For this review, take the finished solid that the model builds, in its own axes (mm). A direction names the side the tool comes from. Give positions to 0.01 mm unless a question says otherwise; leave off trailing zeros. Write each loop counter-clockwise with the first axis right and the second up, starting at its lowest first coordinate (ties: lowest second). Pieces come first, ordered by that corner, then holes.
1) We need section A-A on y = 0. Give the boundary of the cut face in (x, z).
2) We need section C-C on x = 0. Give the boundary of the cut face in (y, z).
3) We need section B-B on z = 5.5. Give the boundary of the cut face in (x, y), and give its area (3 significant figures).
4) For P1, Ø4, axis at y = 63.5, z = 3.5, coming from the -X side, flat-tipped, find the tip position at first contact; note if it passes through.
5) Draft analysis for pull direction Y (two halves, no side actions). For faces 3 (the face through (13, 61, 8)), 4 (the face through (1.35, 6.553, 3.944)), 5 (the face through (8.697, 12.384, 4.056)), 6 (the face through (8.712, -0.744, 3.944)), state which applies: pulls with the +Y half, pulls with the -Y half, needs draft (parallel to the pull), parting line crosses it, or undercut.
6) Machinability: for faces 1 (the face through (-4, 123, 4)), 2 (the face through (1.198, 113.535, 3.944)), which of the approach directions +Z, -Z, +X, -X, +Y, -Y give a long, thin tool a straight path to every point of the face, cutting with its end or side? Answer none if there is none.
7) Wall thickness on line 1 along Y through (x, z) = (-0.25, 5.5) (3 decimals); line 2 along Y through (x, z) = (0, 6.25); line 3 along X through (y, z) = (89, 5.25): over which ranges is each line inside the solid? List them lowest first.
from build123d import *

# Parameters (mm, degrees)
SKETCH_1_R          = 5
EXTRUDE_1_DEPTH     = 8
SKETCH_1_R_2        = 5.001260551
EXTRUDE_1_2_DEPTH   = 8
EXTRUDE_4_DEPTH     = 8
SKETCH_5_R          = 2.5
CUT_EXTRUDE_2_DEPTH = 127.842421926
FILLET_1_R          = 10


with BuildPart() as part:
    # Sketch 1 → Extrude 1 (new body)
    with BuildSketch(Plane.XY):
        with Locations((0, 120)):
            Circle(SKETCH_1_R)
    extrude(amount=EXTRUDE_1_DEPTH)



with BuildPart() as body_2:
    # Sketch 1 → Extrude 1 2 (new body)
    with BuildSketch(Plane.XY):
        Circle(SKETCH_1_R_2)
    extrude(amount=EXTRUDE_1_2_DEPTH)


with BuildPart() as part_1:
    add(part.part)

    add(body_2.part)  # Extrude 4 merges body 2
    # Sketch 4 → Extrude 4 (add)
    with BuildSketch(Plane.XY):
        Polygon((-2.5, 115.669872981), (10, 108.452994616), (10, 11.547005384), (-2.5, 4.330127019), (2.5, -4.330127019), (20, 5.773502692), (20, 114.226497308), (2.5, 124.330127019), align=None)
    extrude(amount=EXTRUDE_4_DEPTH)

    # Sketch 5 → Cut-Extrude 2 (cut, through all)
    with BuildSketch(Plane.XY.offset(8)):
        with Locations((0, 120)):
            Circle(SKETCH_5_R)
        Circle(SKETCH_5_R)
    extrude(amount=-CUT_EXTRUDE_2_DEPTH, mode=Mode.SUBTRACT)

    # Fillet 1
    fillet_1_edges = [part_1.edges().sort_by_distance(p)[0] for p in [
        (10, 11.547005384, 4),
        (20, 5.773502692, 4),
        (20, 114.226497308, 4),
        (10, 108.452994616, 4),
    ]]
    fillet(fillet_1_edges, radius=FILLET_1_R)


solid = part_1.part
Results list:
1. outline: (-5, 0) - (-2.5, 0) - (-2.5, 8) - (-5, 8) - close; (2.5, 0) - (10, 0) - (10, 8) - (2.5, 8) - close
2. outline: (-5, 0) - (-2.5, 0) - (-2.5, 8) - (-5, 8) - close; (2.5, 0) - (5.77, 0) - (5.77, 8) - (2.5, 8) - close; (114.23, 0) - (117.5, 0) - (117.5, 8) - (114.23, 8) - close; (122.5, 0) - (125, 0) - (125, 8) - (122.5, 8) - close
3. outline: (-2.5, 115.67) - (5, 111.34) arc R10 cw to (10, 102.68) - (10, 17.32) arc R10 cw to (5, 8.66) - (-2.4, 4.39) arc R5 ccw (long way) to (2.6, -4.27) - (15, 2.89) arc R10 ccw to (20, 11.55) - (20, 108.45) arc R10 ccw to (15, 117.11) - (2.5, 124.33) arc R5 ccw to start; hole circle Ø5 at (0, 0); hole circle Ø5 at (0, 120)
3. area: 1,410 mm2
4. P1: stops at x = 10
5. face 3: needs draft
5. face 4: undercut
5. face 5: undercut
5. face 6: pulls with the -Y half
6. face 1: +Z, -Z
6. face 2: +Z, -Z, -X
7. line 1: y = -4.995 to -2.487, 2.487 to 5.629, 114.371 to 117.513, 122.487 to 124.994
7. line 2: y = -5 to -2.5, 2.5 to 5.77, 114.23 to 117.5, 122.5 to 125
7. line 3: x = 10 to 20
